Autodesk Inventor part; units mm, degrees
ref_plane "YZ Plane" through (0, 0, 0) normal (1, 0, 0) x (0, 1, 0)
ref_plane "XZ Plane" through (0, 0, 0) normal (0, 1, 0) x (-1, 0, 0)
ref_plane "XY Plane" through (0, 0, 0) normal (0, 0, 1) x (1, 0, 0)
sketch "Sketch1" plane through (0, 0, 0) normal (0, 0, 1) x (1, 0, 0)
  circle A0 centre (0, 0) radius 2
  dimension "Diameter" = 4
extrude "Extrusion1" add sketch "Sketch1" along normal blind 7.52
sketch "Sketch2" plane through (0, 0, 7.52) normal (0, 0, 1) x (1, 0, 0)
  circle A0 centre (0, 0) radius 2
extrude "Extrusion2" add sketch "Sketch2" along normal blind 2.48 draft 45
sketch "Sketch3" plane through (0, 0, 10) normal (0, 0, 1) x (1, 0, 0)
  circle A0 centre (0, 0) radius 4.48
  circle A1 centre (0, 0) radius 1.4434 construction
  line L0 (0.6042, 1.3108) -> (1.4373, 0.1322)
  line L1 (1.4373, 0.1322) -> (0.8331, -1.1787)
  line L2 (0.8331, -1.1787) -> (-0.6042, -1.3108)
  line L3 (-0.6042, -1.3108) -> (-1.4373, -0.1322)
  line L4 (-1.4373, -0.1322) -> (-0.8331, 1.1787)
  line L5 (-0.8331, 1.1787) -> (0.6042, 1.3108)
  dimension "Hex_Width" = 2.5
extrude "Extrusion3" cut sketch "Sketch3" against normal blind 1.5 contours L0 L1 L2 L3 L4 L5
thread "Thread1"
chamfer "Chamfer2" distance 0.4 angle 45 1 edges at (-2, 0, 0)
fillet "Fillet1" radius 0.1 1 edges at (-4.48, 0, 10)
equation "\"d10\" = Thread_Length"
equation "\"d13\" = Chamfer"
equation "\"Thread_Length\" = 7.52"
properties part number "SCREW,FLAT HD,P,12.9,M4X0.7X10MM"
The listing builds one solid part. Answer for the finished solid, in the listing's coordinates (mm). A direction names the side the tool comes from. Give positions to 0.01 mm unless a question says otherwise; leave off trailing zeros. Order: outer loops, then holes, each group sorted by start corner. A loop starts at its lowest first (then second) coordinate and runs counter-clockwise, first axis right, second up. Notation, with made-up numbers: (9.5, -22) -> (22.5, -22) arc R33 cw to (22.5, 11) -> close; hole circle Ø5 at (-3.5, -14.5). An arc over 180 degrees is marked (long way). Answer as CSV lines item,"result". Start each with the question number.
Q1. Find the intervals of material crossed by L1, parallel to X at y = 0, z = 3; L2, parallel to Z at x = 0.75, y = 1; L3, parallel to Y at x = -1, z = 6.25, in increasing order.
Q2. Determine the mould class of faces 3 (the flat face through (0, -2, 10)), 4 (the flat face through (-1.015, -0.73, 9.26)), 5 (the cylindrical face through (0, 2, 4)) for opening direction X: pulls with the +X half, pulls with the -X half, needs draft (parallel to the pull), parting line crosses it, or undercut.
Q3. Given pin 1 (2 mm diameter, centred on x = 2, y = 3, fed in from -Z); pin 2 (2 mm diameter, centred on y = -1.5, z = 5, fed in from +X); pin 3 (1.3 mm diameter, centred on x = 0, y = 0.5, fed in from +Z), each flat-ended and moving along its own axis, determine where each tip first touches the part or whether it passes through.
Q4. A cutting plane is placed at C-C (y = 0). Determine the outline of the cut face in (x, z).
Q5. A cutting plane is placed at A-A (z = 5). Determine the outline of the cut face in (x, y).
Q6. A cutting plane is placed at B-B (x = 0). Determine the outline of the cut face in (y, z), then the cut area to 3 significant figures.
Q7. Which of the six approach directions +Z, -Z, +X, -X, +Y, -Y give full straight-line access (tool end or side, diameter ignored) to faces 1 (the flat face through (0, 0, 8.5)), 2 (the flat face through (0, 0, 0))?
Results found:
1,L1,"-2 to 2"
1,L2,"0 to 8.5"
1,L3,"-1.73 to 1.73"
2,face 3,"needs draft"
2,face 4,"undercut"
2,face 5,"parting line crosses it"
3,pin 1,"z = 8.13"
3,pin 2,"x = 1.94"
3,pin 3,"z = 8.5"
4,outline,"(-4.31, 9.83) -> (-2, 7.52) -> (-2, 0.4) -> (-1.6, 0) -> (1.6, 0) -> (2, 0.4) -> (2, 7.52) -> (4.31, 9.83) arc R0.1 ccw to (4.24, 10) -> (1.38, 10) -> (1.38, 8.5) -> (-1.38, 8.5) -> (-1.38, 10) -> (-4.24, 10) arc R0.1 ccw to start"
5,outline,"circle Ø4 at (0, 0)"
6,outline,"(-4.31, 9.83) -> (-2, 7.52) -> (-2, 0.4) -> (-1.6, 0) -> (1.6, 0) -> (2, 0.4) -> (2, 7.52) -> (4.31, 9.83) arc R0.1 ccw to (4.24, 10) -> (1.26, 10) -> (1.26, 8.5) -> (-1.26, 8.5) -> (-1.26, 10) -> (-4.24, 10) arc R0.1 ccw to start"
6,area,"42.2 mm2"
7,face 1,"+Z"
7,face 2,"-Z, +X, -X, +Y, -Y"
